Autodesk Inventor part; units mm, degrees
ref_plane "YZ Plane" through (0, 0, 0) normal (1, 0, 0) x (0, 1, 0)
ref_plane "XZ Plane" through (0, 0, 0) normal (0, 1, 0) x (-1, 0, 0)
ref_plane "XY Plane" through (0, 0, 0) normal (0, 0, 1) x (1, 0, 0)
sketch "Sketch1" plane through (0, 0, 0) normal (0, 0, 1) x (1, 0, 0)
  line L0 (-50.4258, 38.8802) -> (105.7842, 38.8802)
  line L1 (105.7842, 38.8802) -> (105.7842, 0.7802)
  line L2 (105.7842, 0.7802) -> (-50.4258, 0.7802)
  line L3 (-50.4258, 0.7802) -> (-50.4258, 38.8802)
  line L4 (-122.8158, 267.4802) -> (29.5842, 267.4802)
  line L5 (29.5842, 267.4802) -> (29.5842, 165.8802)
  line L6 (29.5842, 165.8802) -> (-122.8158, 165.8802)
  line L7 (-122.8158, 165.8802) -> (-122.8158, 267.4802)
  line L8 (29.5842, 267.4802) -> (105.7842, 38.8802)
  line L9 (-122.8158, 165.8802) -> (-50.4258, 102.3802)
  line L10 (-50.4258, 102.3802) -> (-50.4258, 38.8802)
  point P0 (0, 0)
  dimension "d0" = 156.21
  dimension "d1" = 38.1
  dimension "d2" = 101.6
  dimension "d3" = 152.4
  dimension "d4" = 228.6
  dimension "d5" = 76.2
  dimension "d19" = 63.5
extrude "Extrusion1" add sketch "Sketch1" along normal blind 19.05
sketch "Sketch5" plane through (0, 0, 0) normal (0, 0, -1) x (-1, 0, 0)
  line L0 (50.4258, 102.3802) -> (50.4258, 0.7802)
  line L1 (122.8158, 165.8802) -> (50.4258, 102.3802)
  line L2 (122.8158, 165.8802) -> (122.8158, 89.6802)
  line L3 (122.8158, 89.6802) -> (50.4258, 26.1802)
  point P0 (0, 0)
  dimension "d40" = 76.2
  dimension "d41" = 76.2
extrude "Extrusion3" add sketch "Sketch5" against normal blind 19.05
sketch "Sketch6" plane through (0, 0, 19.05) normal (0, 0, 1) x (1, 0, 0)
  line L0 (-122.8158, 267.4802) -> (29.5842, 267.4802)
  line L1 (-122.8158, 89.6802) -> (-122.8158, 267.4802)
  point P0 (0, 0)
  point P1 (-72.0158, 216.6802)
  point P2 (-8.5158, 216.6802)
  point P3 (-72.0158, 115.0802)
  point P4 (-72.0158, 165.8802)
  dimension "d44" = 50.8
  dimension "d45" = 50.8
  dimension "d46" = 50.8
  dimension "d47" = 50.8
  dimension "d48" = 50.8
  dimension "d49" = 50.8
  dimension "d50" = 50.8
  dimension "d51" = 63.5
hole "Hole3" at (-72.0158, 216.6802, 19.05) at (-8.5158, 216.6802, 19.05) at (-72.0158, 115.0802, 19.05) at (-72.0158, 165.8802, 19.05) direction (0, 0, -1) diameter 19.05 end through all
fillet "Fillet1" radius 25.4 1 edges at (-50.4258, 26.1802, 9.525)
chamfer "Chamfer1" distance 2.54 angle 45 8 edges at (-8.5158, 226.2052, 0) (-72.0158, 226.2052, 0) (-72.0158, 175.4052, 0) (-72.0158, 124.6052, 0) (-72.0158, 226.2052, 19.05) (-8.5158, 226.2052, 19.05) (-72.0158, 175.4052, 19.05) (-72.0158, 124.6052, 19.05)
properties part number "Uprights"
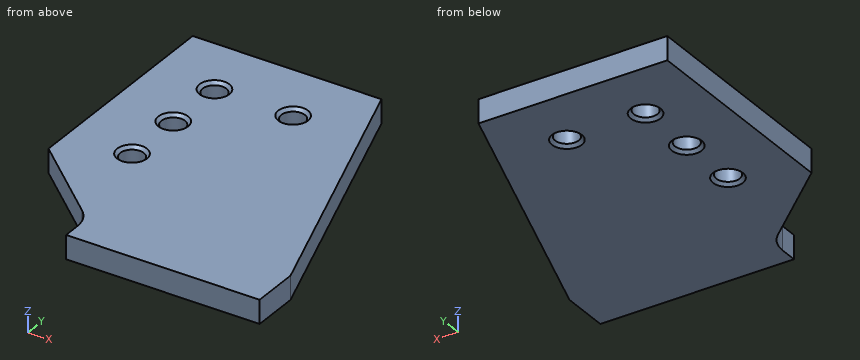
Geometry check sheet. Reference: the model listing, model coordinates, mm. Round coordinates to 2 decimals unless told otherwise and drop trailing zeros. Loops run counter-clockwise (first coordinate to the right, second up) from the corner with the lowest first, then second, coordinate; pieces in that order, holes last. Notation, with made-up numbers: M -34.5,76.5 L 16.5,76.5 A19 ccw 16.5,96.5 Z; hole C -26.75,35 d4. An arc over 180 degrees is marked long. Return JSON: item names as keys, results as strings. Group by question number.
(1) Scan lines: line 1 along X through (y, z) = (214.5, 2.25); line 2 along Y through (x, z) = (-15, 8.5); line 3 along X through (y, z) = (165.5, 8). Record each from-to range of solid material in increasing order. Write a range as [from, to].
(2) Section check B-B, the plane y = 72.5. Enter the section's corners in (x, z).
(3) Section check C-C, the plane x = 46. Enter the section's corners in (y, z), and give its area (3 significant figures).
(4) Go/stop test with flat-tipped pins: pin 1 (1.5 mm diameter, centred on y = 196.5, z = 16.5, fed in from +X); pin 2 (15 mm diameter, centred on x = -72.02, y = 165.88, fed in from -Z); pin 3 (22 mm diameter, centred on x = -8.52, y = 216.68, fed in from -Z); pin 4 (1 mm diameter, centred on y = 116, z = 6.5, fed in from +X). Record where each tip stops, or that it passes through.
(5) Section check A-A, the plane z = 6.5. Enter the section's corners in (x, y) (3 decimals).
Data:
{
 "1": {"line 1": "[-122.82, -81.59], [-62.45, -18.09], [1.05, 47.24]", "line 2": "[0.78, 209.7], [223.66, 267.48]", "line 3": "[-122.82, -81.53], [-62.5, 63.58]"},
 "2": {"outline": "M -103.23,0 L 94.58,0 L 94.58,19.05 L -103.23,19.05 Z"},
 "3": {"outline": "M 0.78,0 L 218.23,0 L 218.23,19.05 L 0.78,19.05 Z", "area": "4,140 mm²"},
 "4": {"pin 1": "x = 53.49", "pin 2": "through", "pin 3": "z = 1.06", "pin 4": "x = 80.24"},
 "5": {"outline": "M -122.816,89.68 L -59.076,33.768 A25.4 cw -50.426,14.673 L -50.426,0.78 L 105.784,0.78 L 105.784,38.88 L 29.584,267.48 L -122.816,267.48 Z; hole C -72.016,115.08 d19.05; hole C -72.016,165.88 d19.05; hole C -72.016,216.68 d19.05; hole C -8.516,216.68 d19.05"}
}
